```python
from build123d import *

# Parameters (mm, degrees)
SKETCH1_W               = 27
SKETCH1_H               = 22
SKETCH1_R               = 1.5
BOSS_EXTRUDE1_DEPTH     = 3
SKETCH2_W               = 5
SKETCH2_H               = 18
BOSS_EXTRUDE2_DEPTH     = 23
CUT_EXTRUDE1_DEPTH      = 33.449961479
CUT_EXTRUDE1_DEPTH_BACK = 33.449961479
SKETCH3_R               = 4
CUT_EXTRUDE2_DEPTH      = 33.449961479
CUT_EXTRUDE2_DEPTH_BACK = 33.449961479
SKETCH4_W               = 9.515030356
SKETCH4_H               = 1.5
FILLET1_R               = 3
FILLET2_R               = 2
FILLET3_R               = 3
SKETCH6_W               = 8
SKETCH6_H               = 8.25
SKETCH6_R               = 2.5
BOSS_EXTRUDE3_DEPTH     = 5
FILLET4_R               = 2


with BuildPart() as part:
    # Sketch1 → Boss-Extrude1 (new body)
    with BuildSketch(Plane.XY):
        Rectangle(SKETCH1_W, SKETCH1_H)
        with Locations((-10.5, -8.5)):
            Circle(SKETCH1_R, mode=Mode.SUBTRACT)
        with Locations((-10.5, 8.5)):
            Circle(SKETCH1_R, mode=Mode.SUBTRACT)
        with Locations((10.5, 8.5)):
            Circle(SKETCH1_R, mode=Mode.SUBTRACT)
        with Locations((10.5, -8.5)):
            Circle(SKETCH1_R, mode=Mode.SUBTRACT)
    extrude(amount=BOSS_EXTRUDE1_DEPTH)

    # Sketch2 → Boss-Extrude2 (add)
    with BuildSketch(Plane.XY.offset(3)):
        Rectangle(SKETCH2_W, SKETCH2_H)
    extrude(amount=BOSS_EXTRUDE2_DEPTH)

    # Sketch3 → Cut-Extrude1 (cut, two sides: drawn at the far end of the back side and taken through both)
    with BuildSketch(Plane(origin=(2.5, 0, 0), x_dir=(0, 0, -1), z_dir=(1, 0, 0)).offset(-CUT_EXTRUDE1_DEPTH_BACK)):
        with Locations(Location((-18, 0, 0), (0, 0, 180))):
            Circle(SKETCH3_R)
    extrude(amount=CUT_EXTRUDE1_DEPTH + CUT_EXTRUDE1_DEPTH_BACK, mode=Mode.SUBTRACT)

    # Sketch4 → Cut-Extrude2 (cut, two sides: drawn at the far end of the back side and taken through both)
    with BuildSketch(Plane(origin=(2.5, 0, 0), x_dir=(0, 0, -1), z_dir=(1, 0, 0)).offset(-CUT_EXTRUDE2_DEPTH_BACK)):
        with Locations((-21.491106051, 0)):
            Rectangle(SKETCH4_W, SKETCH4_H)
    extrude(amount=CUT_EXTRUDE2_DEPTH + CUT_EXTRUDE2_DEPTH_BACK, mode=Mode.SUBTRACT)

    # Fillet1
    fillet1_edges = [part.edges().sort_by_distance(p)[0] for p in [
        (-2.5, 0, 3),
        (2.5, 0, 3),
    ]]
    fillet(fillet1_edges, radius=FILLET1_R)

    # Fillet2
    fillet2_edges = [part.edges().sort_by_distance(p)[0] for p in [
        (0, -9, 3),
        (0, 9, 3),
    ]]
    fillet(fillet2_edges, radius=FILLET2_R - 0.0001)  # a hair under: the kernel refuses the full size

    # Fillet3
    fillet3_edges = [part.edges().sort_by_distance(p)[0] for p in [
        (0, -9, 26),
    ]]
    fillet(fillet3_edges, radius=FILLET3_R)

    # Sketch6 → Boss-Extrude3 (add)
    with BuildSketch(Plane.ZY.offset(2.5)):
        with Locations((30, 4.875)):
            Rectangle(SKETCH6_W, SKETCH6_H)
        with Locations((30, 4.875)):
            Circle(SKETCH6_R, mode=Mode.SUBTRACT)
    extrude(amount=-BOSS_EXTRUDE3_DEPTH)

    # Fillet4
    fillet4_edges = [part.edges().sort_by_distance(p)[0] for p in [
        (0, 0.75, 34),
        (0, 9, 34),
    ]]
    fillet(fillet4_edges, radius=FILLET4_R)


solid = part.part
```
Here's how the part is built. I have some questions about the finished solid (model axes, mm). A direction names the side the tool comes from. Round coordinates to 2 decimals unless told otherwise and drop trailing zeros. Order: outer loops, then holes, each group sorted by start corner. A loop starts at its lowest first (then second) coordinate and runs counter-clockwise, first axis right, second up. Notation, with made-up numbers: (33, 59) -> (66, 59) arc R24 cw to (66, 87) -> close; hole circle Ø1 at (79, 79.5). An arc over 180 degrees is marked (long way). Use a Markdown table: item, result. Add a question column.
(1) Suppose I cut it at B-B, the plane z = 18. Please give me the cut outline in (x, y).
(2) Suppose I cut it at C-C, the plane y = -2.25. Please give me the cut outline in (x, z), and give its area (3 significant figures).
(3) Suppose I cut it at D-D, the plane y = -4.75. Please give me the cut outline in (x, z), and give its area (3 significant figures).
(4) If we mould it in two halves opening along X, with no side actions, what happens to faces 5 (the face through (0, -3, 26)), 6 (the face through (-3.4, 0.15, 3.86)), 7 (the face through (9.3, 7.6, 1.5))? For each: released by +X, released by -X, zero draft, split by the parting line, or undercut.
(5) I need wall thicknesses on line 1 along Y through (x, z) = (-10.5, 2.45); line 2 along Y through (x, z) = (-0.85, 18); line 3 along Y through (x, z) = (-1.35, 30) (3 decimals). Which ranges of each line are inside material? Lowest first, please.
(6) For pin 1 Ø3.5 at (x, z) = (1, 24.5) entering from +Y; pin 2 Ø8 at (y, z) = (-6.5, 20) entering from +X; pin 3 Ø4 at (x, z) = (0.5, 29) entering from -Y, each with a flat end and sliding along its axis, tell me the tip position at first contact or that it passes through.
(7) Suppose I cut it at A-A, the plane x = 10.5. Please give me the cut outline in (y, z).
(8) For faces 1 (the face through (0, -9, 14)), 2 (the face through (2.5, 4.1, 16.7)), 3 (the face through (0, 0.75, 27)), 4 (the face through (-2.5, 4.1, 16.7)), which set-ups out of +Z, -Z, +X, -X, +Y, -Y let a thin tool reach every point of the face, with its end or its side?
Verdict:
| question | item | result |
|---|---|---|
| 1 | outline | (-2.5, -9) -> (2.5, -9) -> (2.5, -4) -> (-2.5, -4) -> close; (-2.5, 4) -> (2.5, 4) -> (2.5, 9) -> (-2.5, 9) -> close |
| 2 | outline | (-13.5, 0) -> (13.5, 0) -> (13.5, 3) -> (5.5, 3) arc R3 cw to (2.5, 6) -> (2.5, 14.69) -> (-2.5, 14.69) -> (-2.5, 6) arc R3 cw to (-5.5, 3) -> (-13.5, 3) -> close; (-2.5, 21.31) -> (2.5, 21.31) -> (2.5, 26) -> (-2.5, 26) -> close |
| 2 | area | 167 mm2 |
| 3 | outline | (-13.5, 0) -> (13.5, 0) -> (13.5, 3) -> (5.5, 3) arc R3 cw to (2.5, 6) -> (2.5, 26) -> (-2.5, 26) -> (-2.5, 6) arc R3 cw to (-5.5, 3) -> (-13.5, 3) -> close |
| 3 | area | 200 mm2 |
| 4 | face 5 | zero draft |
| 4 | face 6 | released by -X |
| 4 | face 7 | undercut |
| 5 | line 1 | -11 to -10, -7 to 7, 10 to 11 |
| 5 | line 2 | -9 to -4, 4 to 9 |
| 5 | line 3 | 0.75 to 2.375, 7.375 to 9 |
| 6 | pin 1 | y = 9 |
| 6 | pin 2 | x = 2.5 |
| 6 | pin 3 | y = 0.75 |
| 7 | outline | (-11, 0) -> (-10, 0) -> (-10, 3) -> (-11, 3) -> close; (-7, 0) -> (7, 0) -> (7, 3) -> (-7, 3) -> close; (10, 0) -> (11, 0) -> (11, 3) -> (10, 3) -> close |
| 8 | face 1 | +Z, +X, -X, -Y |
| 8 | face 2 | +Z, +X, +Y, -Y |
| 8 | face 3 | +Z, +X, -X |
| 8 | face 4 | +Z, -X, +Y, -Y |
